Geometry check sheet. Reference: the model listing, model coordinates, mm. Face numbers are marked on the shaded views. A direction names the side the tool comes from. Round coordinates to 2 decimals unless told otherwise and drop trailing zeros. Order: outer loops, then holes, each group sorted by start corner. A loop starts at its lowest first (then second) coordinate and runs counter-clockwise, first axis right, second up.
(1) Draft check along X on the marked faces 3, 4, 5 and 6. Enter one of: pulls with the +X half, pulls with the -X half, needs draft (parallel to the pull), parting line crosses it, or undercut.
(2) Thickness scan on L1, parallel to X at y = -13.5, z = -22.5; L2, parallel to Y at x = 72.5, z = -0.5; L3, parallel to Y at x = -28, z = -6. Record the ranges inside material, lowest first.
(3) Cross-section at B-B on y = -16.5. Enter the section's corners in (x, z), and give its area (3 significant figures).
(4) Cross-section at D-D on y = -25.5. Enter the section's corners in (x, z), and give its area (3 significant figures).
(5) Cross-section at C-C on x = 31.5. Enter the section's corners in (y, z), and give its area (3 significant figures).
(6) Gauge pin test, flat ends, axial feed: P1, Ø1.5, axis at x = -73, y = -6.5, coming from the +Z side; P2, Ø9.5, axis at x = 27, y = -3.5, coming from the +Z side; P3, Ø2, axis at x = 60, z = -25, coming from the -Y side; P4, Ø10, axis at y = -0.5, z = -28.5, coming from the +X side. Record the tip position at first contact, or that the pin passes through.
(7) Cross-section at A-A on z = -7.5. Enter the section's corners in (x, y).
(8) Set-up check for the marked faces 1 and 2: record each of +Z, -Z, +X, -X, +Y, -Y from which the full face is reachable in a straight line by a thin tool's end or side.
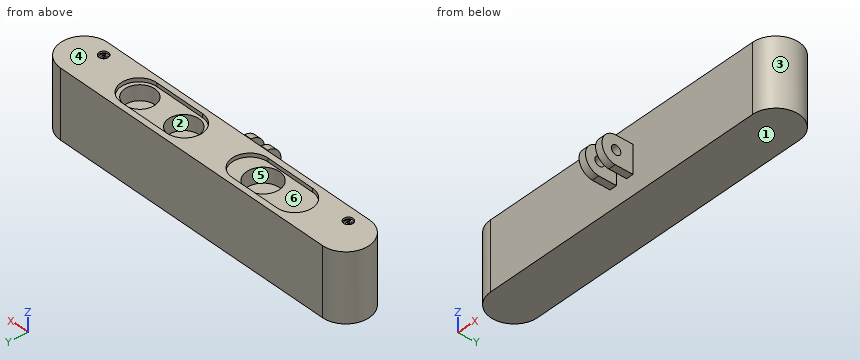
from build123d import *

# Parameters (mm, degrees)
BOSS_EXTRUDE1_DEPTH     = 36
SKETCH3_R               = 8.75
SKETCH3_R_2             = 8
CUT_EXTRUDE1_DEPTH      = 10
CUT_EXTRUDE2_DEPTH      = 2
SKETCH5_R               = 2.5
CUT_EXTRUDE3_DEPTH      = 1
SKETCH6_R               = 0.5
CUT_EXTRUDE4_DEPTH      = 5
SKETCH7_W               = 3.8
SKETCH7_H               = 15
BOSS_EXTRUDE2_DEPTH     = 17
SKETCH8_R               = 2.5
CUT_EXTRUDE5_DEPTH      = 84.2
CUT_EXTRUDE5_DEPTH_BACK = 97.8


with BuildPart() as part:
    # Sketch1 → Boss-Extrude1 (new body)
    with BuildSketch(Plane.XY):
        with BuildLine():
            Line((-77.5, 12.5), (77.5, 12.5))
            ThreePointArc((77.5, 12.5), (90, 0), (77.5, -12.5))
            Line((77.5, -12.5), (-77.5, -12.5))
            ThreePointArc((-77.5, -12.5), (-90, 0), (-77.5, 12.5))
        make_face()
    extrude(amount=-BOSS_EXTRUDE1_DEPTH)

    # Sketch3 → Cut-Extrude1 (cut)
    with BuildSketch(Plane.XY):
        with Locations((-28.5, 0)):
            Circle(SKETCH3_R)
        with Locations((18.5, 0)):
            Circle(SKETCH3_R_2)
        with Locations((44.5, 0)):
            Circle(SKETCH3_R_2)
    extrude(amount=-CUT_EXTRUDE1_DEPTH, mode=Mode.SUBTRACT)

    # Sketch4 → Cut-Extrude2 (cut)
    with BuildSketch(Plane.XY):
        with BuildLine():
            Line((-47.25, 9.5), (-20.75, 9.5))
            ThreePointArc((-20.75, 9.5), (-11.25, 0), (-20.75, -9.5))
            Line((-20.75, -9.5), (-47.25, -9.5))
            ThreePointArc((-47.25, -9.5), (-56.75, 0), (-47.25, 9.5))
        make_face()
        with BuildLine():
            Line((18, 9.5), (45, 9.5))
            ThreePointArc((45, 9.5), (54.5, 0), (45, -9.5))
            Line((45, -9.5), (18, -9.5))
            ThreePointArc((18, -9.5), (8.5, 0), (18, 9.5))
        make_face()
    extrude(amount=-CUT_EXTRUDE2_DEPTH, mode=Mode.SUBTRACT)

    # Sketch5 → Cut-Extrude3 (cut)
    with BuildSketch(Plane.XY):
        with Locations((72.5, -5.85958214)):
            Circle(SKETCH5_R)
        with Locations((-72.5, -5.85958214)):
            Circle(SKETCH5_R)
    extrude(amount=-CUT_EXTRUDE3_DEPTH, mode=Mode.SUBTRACT)

    # Sketch6 → Cut-Extrude4 (cut)
    with BuildSketch(Plane.XY):
        with Locations((-72.5, -5.85958214)):
            Circle(SKETCH6_R)
        with Locations((72.5, -5.85958214)):
            Circle(SKETCH6_R)
        with BuildLine():
            ThreePointArc((-71.394458403, -7.526248807), (-70.5, -5.85958214), (-71.394458403, -4.192915474))
            ThreePointArc((-71.394458403, -4.192915474), (-72.087510469, -4.333196741), (-71.947229202, -5.026248807))
            ThreePointArc((-71.947229202, -5.026248807), (-71.5, -5.85958214), (-71.947229202, -6.692915474))
            ThreePointArc((-71.947229202, -6.692915474), (-72.087510469, -7.385967539), (-71.394458403, -7.526248807))
        make_face()
        with BuildLine():
            ThreePointArc((-73.605541597, -4.192915474), (-74.5, -5.85958214), (-73.605541597, -7.526248807))
            ThreePointArc((-73.605541597, -7.526248807), (-72.912489531, -7.385967539), (-73.052770798, -6.692915474))
            ThreePointArc((-73.052770798, -6.692915474), (-73.5, -5.85958214), (-73.052770798, -5.026248807))
            ThreePointArc((-73.052770798, -5.026248807), (-72.912489531, -4.333196741), (-73.605541597, -4.192915474))
        make_face()
        with BuildLine():
            ThreePointArc((73.605541597, -7.526248807), (74.5, -5.85958214), (73.605541597, -4.192915474))
            ThreePointArc((73.605541597, -4.192915474), (72.912489531, -4.333196741), (73.052770798, -5.026248807))
            ThreePointArc((73.052770798, -5.026248807), (73.5, -5.85958214), (73.052770798, -6.692915474))
            ThreePointArc((73.052770798, -6.692915474), (72.912489531, -7.385967539), (73.605541597, -7.526248807))
        make_face()
        with BuildLine():
            ThreePointArc((71.394458403, -4.192915474), (70.5, -5.85958214), (71.394458403, -7.526248807))
            ThreePointArc((71.394458403, -7.526248807), (72.087510469, -7.385967539), (71.947229202, -6.692915474))
            ThreePointArc((71.947229202, -6.692915474), (71.5, -5.85958214), (71.947229202, -5.026248807))
            ThreePointArc((71.947229202, -5.026248807), (72.087510469, -4.333196741), (71.394458403, -4.192915474))
        make_face()
    extrude(amount=-CUT_EXTRUDE4_DEPTH, mode=Mode.SUBTRACT)

    # Sketch7 → Boss-Extrude2 (add)
    with BuildSketch(Plane.XZ.offset(12.5)):
        with Locations((4.9, -18)):
            Rectangle(SKETCH7_W, SKETCH7_H)
        with Locations((-4.9, -18)):
            Rectangle(SKETCH7_W, SKETCH7_H)
    extrude(amount=BOSS_EXTRUDE2_DEPTH)

    # Sketch8 → Cut-Extrude5 (cut, two sides)
    with BuildSketch(Plane.ZY.offset(6.8)) as cut_extrude5_sk:
        with Locations((-18, -21.484376944)):
            Circle(SKETCH8_R)
        with BuildLine():
            Line((-10.5, -21), (-7.903352706, -21))
            Line((-7.903352706, -21), (-7.606016941, -33.928608258))
            Line((-7.606016941, -33.928608258), (-27.603723976, -34.388521143))
            Line((-27.603723976, -34.388521143), (-27.603723976, -21))
            Line((-27.603723976, -21), (-25.5, -21))
            ThreePointArc((-25.5, -21), (-18, -29.00000207), (-10.5, -21))
        make_face()
    extrude(amount=CUT_EXTRUDE5_DEPTH, mode=Mode.SUBTRACT)
    extrude(cut_extrude5_sk.sketch, amount=-CUT_EXTRUDE5_DEPTH_BACK, mode=Mode.SUBTRACT)


solid = part.part
Found:
1. face 3: pulls with the +X half
1. face 4: needs draft
1. face 5: undercut
1. face 6: undercut
2. L1: x = -6.8 to -3, 3 to 6.8
2. L2: y = -12.5 to -8.36, -3.36 to 12.5
2. L3: y = -12.5 to -8.74, 8.74 to 12.5
3. outline: (-6.8, -25.5) - (-3, -25.5) - (-3, -10.5) - (-6.8, -10.5) - close; (3, -25.5) - (6.8, -25.5) - (6.8, -10.5) - (3, -10.5) - close
3. area: 114 mm2
4. outline: (-6.8, -24.35) - (-3, -24.35) - (-3, -11.65) - (-6.8, -11.65) - close; (3, -24.35) - (6.8, -24.35) - (6.8, -11.65) - (3, -11.65) - close
4. area: 96.6 mm2
5. outline: (-12.5, -36) - (12.5, -36) - (12.5, 0) - (9.5, 0) - (9.5, -2) - (-9.5, -2) - (-9.5, 0) - (-12.5, 0) - close
5. area: 862 mm2
6. P1: stops at z = -1
6. P2: stops at z = -2
6. P3: stops at y = -12.5
6. P4: stops at x = 90
7. outline: (-77.5, -12.5) - (77.5, -12.5) arc R12.5 ccw to (77.5, 12.5) - (-77.5, 12.5) arc R12.5 ccw to start; hole circle Ø17.5 at (-28.5, 0); hole circle Ø16 at (18.5, 0); hole circle Ø16 at (44.5, 0)
8. face 1: -Z, +X, -X, +Y, -Y
8. face 2: +Z
